Build history of the part. All positions in model axes, mm. A direction names the side the tool comes from. Give positions to 0.01 mm unless a question says otherwise; leave off trailing zeros. Order: outer loops, then holes, each group sorted by start corner. A loop starts at its lowest first (then second) coordinate and runs counter-clockwise, first axis right, second up. Notation, with made-up numbers: (52, 87.5) - (101, 87.5) arc R6 ccw to (101, 97.5) - close; hole circle Ø6 at (-14, 6). An arc over 180 degrees is marked (long way). Use a Markdown table: item, result. Add a question column.
(1) Slice it at A-A (x = 16.25). Write the cut outline in (y, z).
(2) Mould opens along X. For faces 4 (the face through (9.664, 2.535, -10.436)), 5 (the face through (23.101, 2.535, -33.305)), 6 (the face through (7.91, 2.6, -39.11)), 7 (the face through (28.71, 2.54, -39.89)) say: +X half, -X half, draft (parallel to the pull), parting line (faces both ways), or undercut.
(3) Which spindle directions (+Z, -Z, +X, -X, +Y, -Y) get a long thin tool onto all of the face, cutting with end or side? Do faces 1 (the face through (3.79, 2.54, -12.11)), 2 (the face through (28.71, 2.54, -13.89)), 3 (the face through (9.156, 2.535, -33.509)). Say none if no direction does.
(4) Slice it at D-D (y = 4.1). Write the cut outline in (x, z) (3 decimals).
(5) Slice it at B-B (z = -32.48). Write the cut outline in (x, y).
(6) Wall check: line 1 (Z direction, x = 24, y = 2.5); line 2 (X direction, y = 2.65, z = -10.07); line 3 (Z direction, x = 23, y = 3.3). Give the ranges that are in metal, low to high.
(7) Slice it at C-C (x = 8.5). Write the cut outline in (y, z).
from build123d import *

# Parameters (mm, degrees)
SKETCH1_W                 = 32.5
SKETCH1_H                 = 52
BOSS_EXTRUDE1_DEPTH       = 5
F_2_56_TAPPED_HOLE1_D     = 1.778
F_2_56_TAPPED_HOLE1_DEPTH = 7.46583491
F_2_56_TAPPED_HOLE1_TIP   = 0.53416509
F_2_56_TAPPED_HOLE2_D     = 1.778
F_2_56_TAPPED_HOLE2_DEPTH = 7.46583491
F_2_56_TAPPED_HOLE2_TIP   = 0.53416509
F_8_32_TAPPED_HOLE1_D     = 3.4544
F_8_32_TAPPED_HOLE1_DEPTH = 9.672193539
F_8_32_TAPPED_HOLE1_TIP   = 1.037806461
SKETCH16_R                = 1.22
CUT_EXTRUDE4_DEPTH        = 5


with BuildPart() as part:
    # Sketch1 → Boss-Extrude1 (new body)
    with BuildSketch(Plane(origin=(0, 0, 0), x_dir=(1, 0, 0), z_dir=(0, 1, 0))):
        with Locations((16.25, 26)):
            Rectangle(SKETCH1_W, SKETCH1_H)
    extrude(amount=BOSS_EXTRUDE1_DEPTH)

    # #2-56 Tapped Hole1
    with Locations(Plane.ZY):
        with Locations((-39, 2.5), (-13, 2.5)):
            Hole(F_2_56_TAPPED_HOLE1_D / 2, depth=F_2_56_TAPPED_HOLE1_DEPTH)
            with Locations((0, 0, -(F_2_56_TAPPED_HOLE1_DEPTH + F_2_56_TAPPED_HOLE1_TIP / 2))):  # 118° drill point
                Cone(0, F_2_56_TAPPED_HOLE1_D / 2, F_2_56_TAPPED_HOLE1_TIP, mode=Mode.SUBTRACT)

    # #2-56 Tapped Hole2
    with Locations(Plane(origin=(32.5, 0, 0), x_dir=(0, 0, -1), z_dir=(1, 0, 0))):
        with Locations((13, 2.5), (39, 2.5)):
            Hole(F_2_56_TAPPED_HOLE2_D / 2, depth=F_2_56_TAPPED_HOLE2_DEPTH)
            with Locations((0, 0, -(F_2_56_TAPPED_HOLE2_DEPTH + F_2_56_TAPPED_HOLE2_TIP / 2))):  # 118° drill point
                Cone(0, F_2_56_TAPPED_HOLE2_D / 2, F_2_56_TAPPED_HOLE2_TIP, mode=Mode.SUBTRACT)

    # #8-32 Tapped Hole1
    with Locations(Plane(origin=(0, 5, 0), x_dir=(1, 0, 0), z_dir=(0, 1, 0))):
        with Locations((16.25, 21.275)):
            Hole(F_8_32_TAPPED_HOLE1_D / 2, depth=F_8_32_TAPPED_HOLE1_DEPTH)
            with Locations((0, 0, -(F_8_32_TAPPED_HOLE1_DEPTH + F_8_32_TAPPED_HOLE1_TIP / 2))):  # 118° drill point
                Cone(0, F_8_32_TAPPED_HOLE1_D / 2, F_8_32_TAPPED_HOLE1_TIP, mode=Mode.SUBTRACT)

    # Sketch16 → Cut-Extrude4 (cut)
    with BuildSketch(Plane(origin=(0, 5, 0), x_dir=(1, 0, 0), z_dir=(0, 1, 0))):
        with Locations((8.5, 32.48)):
            Circle(SKETCH16_R)
        with Locations((24, 32.48)):
            Circle(SKETCH16_R)
        with Locations((8.5, 10.07)):
            Circle(SKETCH16_R)
        with Locations((24, 10.07)):
            Circle(SKETCH16_R)
    extrude(amount=-CUT_EXTRUDE4_DEPTH, mode=Mode.SUBTRACT)


solid = part.part
Solution:
| question | item | result |
|---|---|---|
| 1 | outline | (0, -52) - (5, -52) - (5, -23) - (0, -23) - close; (0, -19.55) - (5, -19.55) - (5, 0) - (0, 0) - close |
| 2 | face 4 | undercut |
| 2 | face 5 | undercut |
| 2 | face 6 | -X half |
| 2 | face 7 | draft |
| 3 | face 1 | -X |
| 3 | face 2 | +X |
| 3 | face 3 | +Y, -Y |
| 4 | outline | (0, -52) - (32.5, -52) - (32.5, 0) - (0, 0) - close; hole circle Ø2.44 at (8.5, -32.48); hole circle Ø2.44 at (8.5, -10.07); hole circle Ø3.454 at (16.25, -21.275); hole circle Ø2.44 at (24, -32.48); hole circle Ø2.44 at (24, -10.07) |
| 5 | outline | (0, 0) - (7.28, 0) - (7.28, 5) - (0, 5) - close; (9.72, 0) - (22.78, 0) - (22.78, 5) - (9.72, 5) - close; (25.22, 0) - (32.5, 0) - (32.5, 5) - (25.22, 5) - close |
| 6 | line 1 | -52 to -33.7, -31.26 to -11.29, -8.85 to 0 |
| 6 | line 2 | 0 to 7.28, 9.72 to 22.78, 25.22 to 32.5 |
| 6 | line 3 | -52 to -33.18, -31.78 to -10.77, -9.37 to 0 |
| 7 | outline | (0, -52) - (5, -52) - (5, -33.7) - (0, -33.7) - close; (0, -31.26) - (5, -31.26) - (5, -11.29) - (0, -11.29) - close; (0, -8.85) - (5, -8.85) - (5, 0) - (0, 0) - close |
